```python
from build123d import *

# Parameters (mm, degrees)
F0_W     = 81.613116
F0_H     = 21.423442
F1_DEPTH = 25.4
F2_SIZE  = 5.08
F3_R     = 5.08


with BuildPart() as f1:
    # F0 (on Top) → F1 (new body)
    with BuildSketch(Plane.XY):
        with Locations((40.806558, 10.711721)):
            Rectangle(F0_W, F0_H)
    extrude(amount=F1_DEPTH)

    # F2
    f2_edges = [f1.edges().sort_by_distance(p)[0] for p in [
        (0, 10.711721, 25.4),
        (0, 21.423442, 12.7),
        (0, 0, 12.7),
        (0, 10.711721, 0),
    ]]
    chamfer(f2_edges, length=F2_SIZE)

    # F3
    f3_edges = [f1.edges().sort_by_distance(p)[0] for p in [
        (81.613116, 0, 12.7),
        (81.613116, 21.423442, 12.7),
        (81.613116, 10.711721, 0),
        (81.613116, 10.711721, 25.4),
    ]]
    fillet(f3_edges, radius=F3_R)


solid = f1.part
```
Input: part model. Units: mm. Frame: model coordinates. Coordinates: 2 decimals unless noted, no trailing zeros. Order: outer loops, then holes, each group sorted by start corner. A loop starts at its lowest first (then second) coordinate and runs counter-clockwise, first axis right, second up. Notation, with made-up numbers: (4, -25) - (11, -25) arc R31 cw to (11, 9) - close; hole circle Ø1 at (83.25, 20.5). An arc over 180 degrees is marked (long way). Put each result on its own line as item: value.
1. Cut plane A-A on y = 9.25. Return the cut outline in (x, z).
Report:
outline: (0, 5.08) - (5.08, 0) - (76.53, 0) arc R5.08 ccw to (81.61, 5.08) - (81.61, 20.32) arc R5.08 ccw to (76.53, 25.4) - (5.08, 25.4) - (0, 20.32) - close
2. Cut plane B-B on z = 13.25. Return the cut outline in (x, y).
Report:
outline: (0, 5.08) - (5.08, 0) - (76.53, 0) arc R5.08 ccw to (81.61, 5.08) - (81.61, 16.34) arc R5.08 ccw to (76.53, 21.42) - (5.08, 21.42) - (0, 16.34) - close
3. Line query: line 1 along X through (y, z) = (2.25, 15.25); line 2 along Y through (x, z) = (4, 9.5); line 3 along X through (y, z) = (19, 20.75). Output: solid intervals per line, ascending.
Report:
line 1: x = 2.83 to 80.75
line 2: y = 1.08 to 20.34
line 3: x = 2.66 to 80.86
